Geometry check sheet. Reference: the model listing, model coordinates, mm. A direction names the side the tool comes from. Give positions to 0.01 mm unless a question says otherwise; leave off trailing zeros. Loops run counter-clockwise (first coordinate to the right, second up) from the corner with the lowest first, then second, coordinate; pieces in that order, holes last.
```python
from build123d import *

# Parameters (mm, degrees)
SKETCH1_R                = 14.975
SKETCH1_R_2              = 9.975
BOSS_EXTRUDE1_DEPTH      = 25
BOSS_EXTRUDE2_DEPTH      = 5.5
BOSS_EXTRUDE2_DEPTH_BACK = 5.5
SKETCH2_R                = 20.75
SKETCH2_R_2              = 9.975


with BuildPart() as part:
    # Sketch1 → Boss-Extrude1 (new body)
    with BuildSketch(Plane(origin=(0, 0, 0), x_dir=(0, 0, -1), z_dir=(1, 0, 0))):
        Circle(SKETCH1_R)
        Circle(SKETCH1_R_2, mode=Mode.SUBTRACT)
    extrude(amount=BOSS_EXTRUDE1_DEPTH)

    # Sketch2 → Boss-Extrude2 (add, two sides: drawn at the far end of the back side and taken through both)
    with BuildSketch(Plane(origin=(12.5, 0, 0), x_dir=(0, 0, -1), z_dir=(1, 0, 0)).offset(-BOSS_EXTRUDE2_DEPTH_BACK)):
        Circle(SKETCH2_R)
        Circle(SKETCH2_R_2, mode=Mode.SUBTRACT)
    extrude(amount=BOSS_EXTRUDE2_DEPTH + BOSS_EXTRUDE2_DEPTH_BACK)


solid = part.part
```
1) Depth check by flat-ended pin: P1, Ø3, axis at y = -15.5, z = 1, coming from the -X side; P2, Ø1.5, axis at x = 8, y = -6, coming from the -Z side; P3, Ø10, axis at x = 8, z = 8, coming from the +Y side; P4, Ø6, axis at x = 11.5, z = -2.5, coming from the -Y side. Enter the tip coordinate at first touch or a pass-through.
2) Sectioned sample at A-A on z = 0. Enter the section's corners in (x, y) (3 decimals), plus the area to 3 significant figures.
3) Scan lines: line 1 along Y through (x, z) = (7.25, -0.5); line 2 along Y through (x, z) = (15.75, 4.5). Record each from-to range of solid material in increasing order.
4) Mould release check, pull along Z, two halves, no side actions. Record for faces 1 (the cylindrical face through (12.4, 6.2, -19.8)), 2 (the flat face through (0, -3, -10)), 3 (the cylindrical face through (12.325, 2.996, -9.514)): +Z half, -Z half, draft (parallel to the pull), parting line (faces both ways), or undercut.
5) Sectioned sample at C-C on y = 11. Enter the section's corners in (x, z), plus the area to 3 significant figures.
6) Sectioned sample at D-D on x = 17. Enter the section's corners in (y, z) (3 decimals), plus the area to 3 significant figures.
7) Tool access check on faces 4 (the flat face through (18, -14, -6)), 5 (the flat face through (7, -14, -6)), 6 (the flat face through (25, -3, -10)). Record the directions out of +Z, -Z, +X, -X, +Y, -Y that give a thin tool (end or side, any length) a straight path to the whole face; none if there is none.
Determined:
1. P1: stops at x = 0
1. P2: stops at z = -20.07
1. P3: stops at y = 20.53
1. P4: stops at y = -20.75
2. outline: (0, -14.975) - (7, -14.975) - (7, -20.75) - (18, -20.75) - (18, -14.975) - (25, -14.975) - (25, -9.975) - (0, -9.975) - close; (0, 9.975) - (25, 9.975) - (25, 14.975) - (18, 14.975) - (18, 20.75) - (7, 20.75) - (7, 14.975) - (0, 14.975) - close
2. area: 377 mm2
3. line 1: y = -20.74 to -9.96, 9.96 to 20.74
3. line 2: y = -20.26 to -8.9, 8.9 to 20.26
4. face 1: parting line
4. face 2: draft
4. face 3: undercut
5. outline: (0, -10.16) - (7, -10.16) - (7, -17.59) - (18, -17.59) - (18, -10.16) - (25, -10.16) - (25, 10.16) - (18, 10.16) - (18, 17.59) - (7, 17.59) - (7, 10.16) - (0, 10.16) - close
5. area: 672 mm2
6. outline: circle Ø41.5 at (0, 0); hole circle Ø19.95 at (0, 0)
6. area: 1,040 mm2
7. face 4: +X
7. face 5: -X
7. face 6: +Z, -Z, +X, +Y, -Y
